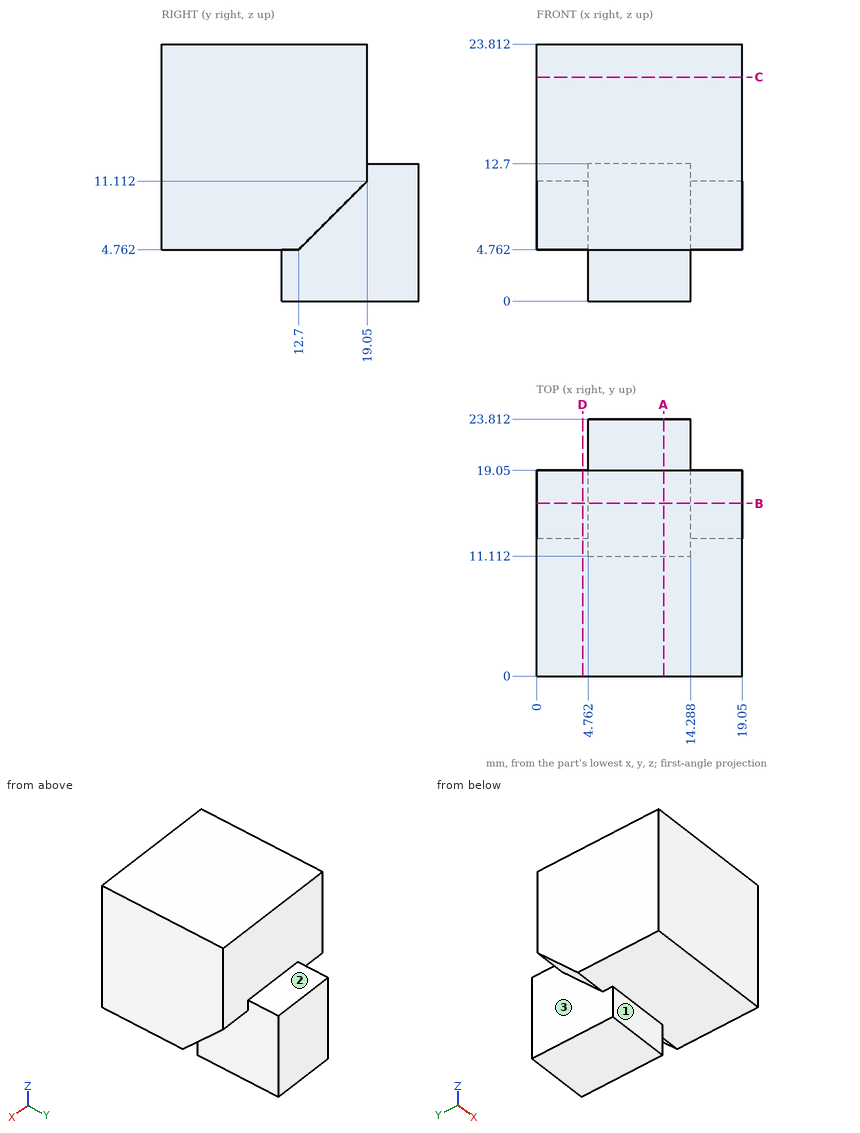
Print and shaded views of the part. All mm, measured from the part's lowest x, y and z. A direction names the side the tool comes from. Coordinates: 2 decimals unless noted, no trailing zeros. Order: outer loops, then holes, each group sorted by start corner. A loop starts at its lowest first (then second) coordinate and runs counter-clockwise, first axis right, second up. Notation, with made-up numbers: (25.25, 11) -> (47.25, 11) arc R28 ccw to (47.25, 44) -> close; hole circle Ø8 at (-36, -31). An arc over 180 degrees is marked (long way). Answer as a JSON object with one key per item and string values. Group by question number.
1) Cut at C-C, the plane z = 20.75. Write the cut outline in (x, y), then the cut area to 3 significant figures.
2) Drill centre lines: L1, parallel to Z at x = 8.25, y = 19.5; L2, parallel to Z at x = 3, y = 2.5; L3, parallel to Y at x = 16.25, z = 13.25. Where is each one in solid material? Low to high.
3) Flat gauge pins, fed straight in: pin 1 (14 mm diameter, centred on y = 14.5, z = 6.5, fed in from +X); pin 2 (5 mm diameter, centred on x = 9, z = 2, fed in from -Y); pin 3 (8 mm diameter, centred on x = 7.5, y = 6.5, fed in from -Z); pin 4 (2 mm diameter, centred on x = 7, z = 18, fed in from +Y). Where does each tip first touch, or does it go through?
4) Cut at A-A, the plane x = 11.75. Write the cut outline in (y, z), then the cut area to 3 significant figures.
5) Cut at B-B, the plane y = 16. Write the cut outline in (x, z).
6) Which spindle directions (+Z, -Z, +X, -X, +Y, -Y) get a long thin tool onto all of the face, cutting with end or side? Do the marked faces 1, 2 and 3. Say none if no direction does.
7) Cut at D-D, the plane x = 4.25. Write the cut outline in (y, z).
Check values:
{
 "1": {"outline": "(0, 0) -> (19.05, 0) -> (19.05, 19.05) -> (0, 19.05) -> close", "area": "363 mm²"},
 "2": {"L1": "z = 0 to 12.7", "L2": "z = 4.76 to 23.81", "L3": "y = 0 to 19.05"},
 "3": {"pin 1": "stops at x = 19.05", "pin 2": "stops at y = 11.11", "pin 3": "stops at z = 4.76", "pin 4": "stops at y = 19.05"},
 "4": {"outline": "(0, 4.76) -> (11.11, 4.76) -> (11.11, 0) -> (23.81, 0) -> (23.81, 12.7) -> (19.05, 12.7) -> (19.05, 23.81) -> (0, 23.81) -> close", "area": "461 mm²"},
 "5": {"outline": "(0, 8.06) -> (4.76, 8.06) -> (4.76, 0) -> (14.29, 0) -> (14.29, 8.06) -> (19.05, 8.06) -> (19.05, 23.81) -> (0, 23.81) -> close"},
 "6": {"face 1": "-Z, +X, -X, -Y", "face 2": "+Z, +X, -X, +Y", "face 3": "-Z, -X, +Y"},
 "7": {"outline": "(0, 4.76) -> (12.7, 4.76) -> (19.05, 11.11) -> (19.05, 23.81) -> (0, 23.81) -> close"}
}
